Design review of the part built by this model. Coordinates are the model's own, in mm. Face numbers are marked on the shaded views. A direction names the side the tool comes from. Give positions to 0.01 mm unless a question says otherwise; leave off trailing zeros. Write each loop counter-clockwise with the first axis right and the second up, starting at its lowest first coordinate (ties: lowest second). Pieces come first, ordered by that corner, then holes.
```python
from build123d import *

# Parameters (mm, degrees)
PAD045_DEPTH         = 15
SKETCH178_R          = 8.4
POCKET110_DEPTH      = 40.078905
SKETCH180_R          = 3.25
POCKET111_DEPTH      = 4.001
SKETCH181_R          = 62.5
SKETCH181_R_2        = 20
POCKET112_DEPTH      = 14.001
POCKET112_DEPTH_BACK = 30.078905
SKETCH183_R          = 2.2
POCKET114_DEPTH      = 15.001
POCKET114_DEPTH_BACK = 15.001
SKETCH184_W          = 6
SKETCH184_H          = 53.327905
POCKET193_DEPTH      = 15.001
POCKET193_DEPTH_BACK = 15.001
SKETCH286_R          = 2.8
POCKET194_DEPTH      = 4
CHAMFER004_SIZE      = 0.4


with BuildPart() as part:
    # Sketch177 → Pad045 (new body, symmetric)
    with BuildSketch(Plane.XZ):
        Polygon((-18, -14), (15, 19), (15, 30.077905), (-20, 30.077905), (-20, -14), align=None)
    extrude(amount=PAD045_DEPTH, both=True)

    # Sketch178 (on DatumPlane) → Pocket110 (cut, through all)
    with BuildSketch(Plane.XY.offset(26.077905)):
        Circle(SKETCH178_R)
    extrude(amount=-POCKET110_DEPTH, mode=Mode.SUBTRACT)

    # Sketch180 (on DatumPlane) → Pocket111 (cut, through all)
    with BuildSketch(Plane.XY.offset(26.077905)):
        Circle(SKETCH180_R)
    extrude(amount=POCKET111_DEPTH, mode=Mode.SUBTRACT)

    # Sketch181 → Pocket112 (cut, two sides)
    with BuildSketch(Plane.XY) as pocket112_sk:
        Circle(SKETCH181_R)
        Circle(SKETCH181_R_2, mode=Mode.SUBTRACT)
    extrude(amount=-POCKET112_DEPTH, mode=Mode.SUBTRACT)
    extrude(pocket112_sk.sketch, amount=POCKET112_DEPTH_BACK, mode=Mode.SUBTRACT)

    # Sketch183 → Pocket114 (cut, two sides)
    with BuildSketch(Plane.XZ) as pocket114_sk:
        with Locations((0, 14)):
            Circle(SKETCH183_R)
    extrude(amount=-POCKET114_DEPTH, mode=Mode.SUBTRACT)
    extrude(pocket114_sk.sketch, amount=POCKET114_DEPTH_BACK, mode=Mode.SUBTRACT)

    # Sketch184 → Pocket193 (cut, two sides)
    with BuildSketch(Plane.XZ) as pocket193_sk:
        with Locations((-18, -4.586048)):
            Rectangle(SKETCH184_W, SKETCH184_H)
    extrude(amount=-POCKET193_DEPTH, mode=Mode.SUBTRACT)
    extrude(pocket193_sk.sketch, amount=POCKET193_DEPTH_BACK, mode=Mode.SUBTRACT)

    # Sketch286 (on Face7 of Pad045) → Pocket194 (cut)
    with BuildSketch(Plane.XZ.offset(15)):
        with Locations((0, 14)):
            Circle(SKETCH286_R)
    pocket194 = extrude(amount=-POCKET194_DEPTH, mode=Mode.SUBTRACT)

    # Mirrored010: Pocket194 across XZ
    add(pocket194.mirror(Plane.XZ), mode=Mode.SUBTRACT)

    # Chamfer004
    chamfer004_edges = [part.edges().sort_by_distance(p)[0] for p in [
        (-18.228757, 8.228757, 30.077905),
        (-18.228757, -8.228757, 30.077905),
        (0, 15, 30.077905),
        (14.142136, 14.142136, 30.077905),
        (15, 0, 30.077905),
        (14.142136, -14.142136, 30.077905),
        (0, -15, 30.077905),
        (15, 0, 19),
        (14.132889, 14.151376, 18.132889),
        (0, 15, 4),
        (14.132889, -14.151376, 18.132889),
        (0, -15, 4),
        (-8.399998, -0.005359, -4.399998),
        (-14.132889, 14.151376, -10.132889),
        (-15, 0, -11),
        (-14.132889, -14.151376, -10.132889),
        (-18.708287, -7.071068, 22.077905),
        (-18.708287, 7.071068, 22.077905),
    ]]
    chamfer(chamfer004_edges, length=CHAMFER004_SIZE)


with BuildPart() as part_1:
    # Body022036 placement: moved
    add(part.part.moved(Location((-3.125, 0, 854.79899))))


solid = part_1.part
```
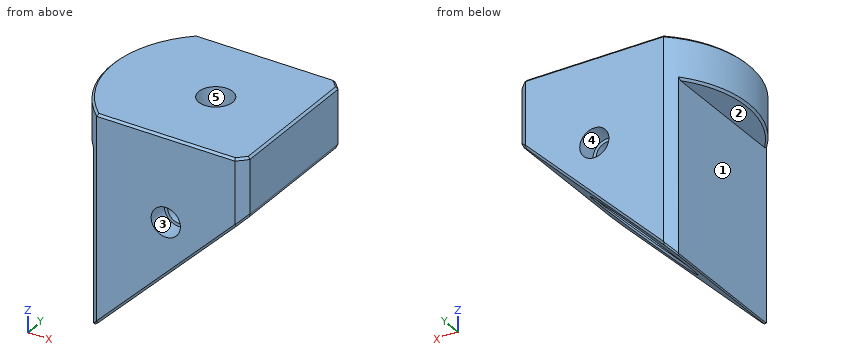
(1) Tool access review of the marked faces 4 and 5: name each direction out of +Z, -Z, +X, -X, +Y, -Y from which nothing blocks a thin tool from reaching the whole face with its end or side.
Resolved:
face 4: +Y
face 5: +Z, -Z
(2) To check wall thickness, follow L1, parallel to X at y = 0, z = 882.4 (3 decimals); L2, parallel to Z at x = 0, y = -1; L3, parallel to Y at x = -5.5, z = 865.5. State the ranges of each line that lie inside material, in increasing order.
Resolved:
L1: x = -23.125 to -6.375, 0.125 to 11.875
L2: z = 880.88 to 884.88
L3: y = -15 to -8.06, 8.06 to 15
(3) Consider section A-A, the plane x = 6.5. Give the boundary of the cut face in (y, z), then the cut area to 3 significant figures.
Resolved:
outline: (-15, 868.99) - (-14.6, 868.42) - (14.6, 868.42) - (15, 868.99) - (15, 884.48) - (14.6, 884.88) - (-14.6, 884.88) - (-15, 884.48) - close
area: 493 mm2
(4) Mouldability with a two-part tool opening along X and no side actions: class the marked faces 1, 2 and 3 as pulls with the +X half, pulls with the -X half, needs draft (parallel to the pull), parting line crosses it, or undercut.
Resolved:
face 1: pulls with the -X half
face 2: needs draft
face 3: undercut
(5) Clearance check with flat-ended pins moving along their axes: P1, Ø1, axis at y = 2.5, z = 858, coming from the -X side (3 decimals); P2, Ø1, axis at y = 9.5, z = 859, coming from the +X side; P3, Ø8.5, axis at x = -1.5, y = -3, coming from the -Z side. State where each tip first meets the part, or that it passes through.
Resolved:
P1: stops at x = -18.125
P2: stops at x = -2.42
P3: stops at z = 880.88
